Input: part model. Units: mm. Frame: model coordinates. A direction names the side the tool comes from. Round coordinates to 2 decimals unless told otherwise and drop trailing zeros. Loops run counter-clockwise (first coordinate to the right, second up) from the corner with the lowest first, then second, coordinate; pieces in that order, holes last. Notation, with made-up numbers: M -11.5,12.5 L 16.5,12.5 A31 cw 16.5,49.5 Z; hole C 41.5,25 d8. An arc over 180 degrees is marked long. Put each result on its own line as item: value. Start each with the question number.
1) Line query: probe 1 along Y at (x, z) = (0.7, -29); probe 2 along Y at (x, z) = (2.3, 20). Output: solid intervals per line, ascending.
2) Draft query along Y for faces 3 (the face through (1, -24, 0)), 4 (the face through (1.52, -27, -31.45)), 5 (the face through (1, 0, -32.5)), 6 (the face through (2.507, -12.307, 18.8)). Return one class per face: +Y half, -Y half, draft (parallel to the pull), parting line (faces both ways), or undercut.
3) Reachability of faces 1 (the face through (1, 6, 27.857)), 2 (the face through (7, 22.99, 29.05)) from +Z, -Z, +X, -X, +Y, -Y: full face, straight path, thin tool, end or side. Return the list, or none.
4) Section C-C on z = -1. Output: boundary loops of the cut face in (x, y), plus the area to 3 significant figures.
5) Section B-B on y = -10. Output: boundary loops of the cut face in (x, z).
6) Section D-D on z = -20. Output: boundary loops of the cut face in (x, y), plus the area to 3 significant figures.
7) Pin query (flat end, axial travel): pin 1 (1.6 mm diameter, centred on y = -9.5, z = 19, fed in from +X); pin 2 (1.8 mm diameter, centred on y = -19.5, z = 21.5, fed in from +X). Return the tip coordinate at first contact, or that it passes through.
from build123d import *
from build123d.topology import SkipClean

# Parameters (mm, degrees)
SKETCH1_W           = 65
SKETCH1_H           = 56
SKETCH1_W_2         = 55.714285714
SKETCH1_H_2         = 48
BOSS_EXTRUDE1_DEPTH = 3
BOSS_EXTRUDE2_DEPTH = 4
BOSS_EXTRUDE3_DEPTH = 3
SKETCH4_R           = 1.35
CUT_EXTRUDE1_DEPTH  = 44.084219849
FILLET1_R           = 3.5
SKETCH5_W           = 55.714285714
SKETCH5_H           = 10
BOSS_EXTRUDE4_DEPTH = 3
SKETCH6_R           = 1.3
CUT_EXTRUDE2_DEPTH  = 44.084219849
BOSS_EXTRUDE5_DEPTH = 3
SKETCH8_R           = 2.6
CUT_EXTRUDE3_DEPTH  = 1


with BuildPart() as part:
    # Sketch1 → Boss-Extrude1 (new body)
    with BuildSketch(Plane(origin=(0, 0, 0), x_dir=(0, 0, -1), z_dir=(1, 0, 0))):
        Rectangle(SKETCH1_W, SKETCH1_H)
        Rectangle(SKETCH1_W_2, SKETCH1_H_2, mode=Mode.SUBTRACT)
    extrude(amount=BOSS_EXTRUDE1_DEPTH)

    # Sketch2 → Boss-Extrude2 (add)
    with BuildSketch(Plane(origin=(3, 0, 0), x_dir=(0, 0, -1), z_dir=(1, 0, 0))):
        with BuildLine():
            ThreePointArc((-25.5, 24.5), (-31.474873734, 26.974873734), (-29, 21))
            Line((-29, 21), (-29, 23.15))
            ThreePointArc((-29, 23.15), (-29.954594155, 25.454594155), (-27.65, 24.5))
            Line((-27.65, 24.5), (-25.5, 24.5))
        make_face()
        with BuildLine():
            Line((-29, 23.15), (-29, 21))
            ThreePointArc((-29, 21), (-28.420576225, 21.048294901), (-27.857142857, 21.191846807))
            Line((-27.857142857, 21.191846807), (-27.857142857, 23.781405851))
            ThreePointArc((-27.857142857, 23.781405851), (-28.347160855, 23.318348169), (-29, 23.15))
        make_face()
        with BuildLine():
            Line((-27.857142857, 23.781405851), (-27.857142857, 21.191846807))
            ThreePointArc((-27.857142857, 21.191846807), (-26.302325383, 22.270078104), (-25.535898385, 24))
            Line((-25.535898385, 24), (-27.74600638, 24))
            ThreePointArc((-27.74600638, 24), (-27.796600962, 23.888174245), (-27.857142857, 23.781405851))
        make_face()
        with BuildLine():
            ThreePointArc((-25.535898385, 24), (-25.508986132, 24.249356481), (-25.5, 24.5))
            Line((-25.5, 24.5), (-27.65, 24.5))
            ThreePointArc((-27.65, 24.5), (-27.674218836, 24.245433101), (-27.74600638, 24))
            Line((-27.74600638, 24), (-25.535898385, 24))
        make_face()
        with BuildLine():
            Line((29, 23.15), (29, 21))
            ThreePointArc((29, 21), (31.474873734, 22.025126266), (32.5, 24.5))
            ThreePointArc((32.5, 24.5), (29, 28), (25.5, 24.5))
            Line((25.5, 24.5), (27.65, 24.5))
            ThreePointArc((27.65, 24.5), (29, 25.85), (30.35, 24.5))
            ThreePointArc((30.35, 24.5), (29.954594155, 23.545405845), (29, 23.15))
        make_face()
        with BuildLine():
            Line((27.65, 24.5), (25.5, 24.5))
            ThreePointArc((25.5, 24.5), (25.508986132, 24.249356481), (25.535898385, 24))
            Line((25.535898385, 24), (27.74600638, 24))
            ThreePointArc((27.74600638, 24), (27.674218836, 24.245433101), (27.65, 24.5))
        make_face()
        with BuildLine():
            ThreePointArc((25.535898385, 24), (26.302325383, 22.270078104), (27.857142857, 21.191846807))
            Line((27.857142857, 21.191846807), (27.857142857, 23.781405851))
            ThreePointArc((27.857142857, 23.781405851), (27.796600962, 23.888174245), (27.74600638, 24))
            Line((27.74600638, 24), (25.535898385, 24))
        make_face()
        with BuildLine():
            Line((27.857142857, 23.781405851), (27.857142857, 21.191846807))
            ThreePointArc((27.857142857, 21.191846807), (28.420576225, 21.048294901), (29, 21))
            Line((29, 21), (29, 23.15))
            ThreePointArc((29, 23.15), (28.347160855, 23.318348169), (27.857142857, 23.781405851))
        make_face()
        with BuildLine():
            Line((27.65, -24.5), (25.5, -24.5))
            ThreePointArc((25.5, -24.5), (29, -28), (32.5, -24.5))
            ThreePointArc((32.5, -24.5), (31.474873734, -22.025126266), (29, -21))
            Line((29, -21), (29, -23.15))
            ThreePointArc((29, -23.15), (29.954594155, -23.545405845), (30.35, -24.5))
            ThreePointArc((30.35, -24.5), (29, -25.85), (27.65, -24.5))
        make_face()
        with BuildLine():
            ThreePointArc((29, -21), (28.420576225, -21.048294901), (27.857142857, -21.191846807))
            Line((27.857142857, -21.191846807), (27.857142857, -23.781405851))
            ThreePointArc((27.857142857, -23.781405851), (28.347160855, -23.318348169), (29, -23.15))
            Line((29, -23.15), (29, -21))
        make_face()
        with BuildLine():
            ThreePointArc((27.857142857, -21.191846807), (26.302325383, -22.270078104), (25.535898385, -24))
            Line((25.535898385, -24), (27.74600638, -24))
            ThreePointArc((27.74600638, -24), (27.796600962, -23.888174245), (27.857142857, -23.781405851))
            Line((27.857142857, -23.781405851), (27.857142857, -21.191846807))
        make_face()
        with BuildLine():
            ThreePointArc((25.535898385, -24), (25.508986132, -24.249356481), (25.5, -24.5))
            Line((25.5, -24.5), (27.65, -24.5))
            ThreePointArc((27.65, -24.5), (27.674218836, -24.245433101), (27.74600638, -24))
            Line((27.74600638, -24), (25.535898385, -24))
        make_face()
        with BuildLine():
            ThreePointArc((-29, -21), (-31.474873734, -26.974873734), (-25.5, -24.5))
            Line((-25.5, -24.5), (-27.65, -24.5))
            ThreePointArc((-27.65, -24.5), (-29.954594155, -25.454594155), (-29, -23.15))
            Line((-29, -23.15), (-29, -21))
        make_face()
        with BuildLine():
            ThreePointArc((-27.857142857, -21.191846807), (-28.420576225, -21.048294901), (-29, -21))
            Line((-29, -21), (-29, -23.15))
            ThreePointArc((-29, -23.15), (-28.347160855, -23.318348169), (-27.857142857, -23.781405851))
            Line((-27.857142857, -23.781405851), (-27.857142857, -21.191846807))
        make_face()
        with BuildLine():
            Line((-27.74600638, -24), (-25.535898385, -24))
            ThreePointArc((-25.535898385, -24), (-26.302325383, -22.270078104), (-27.857142857, -21.191846807))
            Line((-27.857142857, -21.191846807), (-27.857142857, -23.781405851))
            ThreePointArc((-27.857142857, -23.781405851), (-27.796600962, -23.888174245), (-27.74600638, -24))
        make_face()
        with BuildLine():
            Line((-27.65, -24.5), (-25.5, -24.5))
            ThreePointArc((-25.5, -24.5), (-25.508986132, -24.249356481), (-25.535898385, -24))
            Line((-25.535898385, -24), (-27.74600638, -24))
            ThreePointArc((-27.74600638, -24), (-27.674218836, -24.245433101), (-27.65, -24.5))
        make_face()
    extrude(amount=BOSS_EXTRUDE2_DEPTH)

    # Sketch3 → Boss-Extrude3 (add)
    with SkipClean():  # the faces are left unmerged after this step: merging them gives an invalid solid
        with BuildSketch(Plane.ZY):
            with BuildLine():
                Line((-27.74600638, 24), (-27.857142857, 24))
                Line((-27.857142857, 24), (-27.857142857, 23.781405851))
                Line((-27.857142857, 23.781405851), (-27.857142857, 21.191846807))
                ThreePointArc((-27.857142857, 21.191846807), (-26.302325383, 22.270078104), (-25.535898385, 24))
                Line((-25.535898385, 24), (-27.74600638, 24))
            make_face()
            with BuildLine():
                Line((27.857142857, 21.191846807), (27.857142857, 23.781405851))
                Line((27.857142857, 23.781405851), (27.857142857, 24))
                Line((27.857142857, 24), (27.74600638, 24))
                Line((27.74600638, 24), (25.535898385, 24))
                ThreePointArc((25.535898385, 24), (26.302325383, 22.270078104), (27.857142857, 21.191846807))
            make_face()
            with BuildLine():
                Line((-27.857142857, -21.191846807), (-27.857142857, -23.781405851))
                Line((-27.857142857, -23.781405851), (-27.857142857, -24))
                Line((-27.857142857, -24), (-27.74600638, -24))
                Line((-27.74600638, -24), (-25.535898385, -24))
                ThreePointArc((-25.535898385, -24), (-26.302325383, -22.270078104), (-27.857142857, -21.191846807))
            make_face()
            with BuildLine():
                Line((27.857142857, -23.781405851), (27.857142857, -21.191846807))
                ThreePointArc((27.857142857, -21.191846807), (26.302325383, -22.270078104), (25.535898385, -24))
                Line((25.535898385, -24), (27.74600638, -24))
                Line((27.74600638, -24), (27.857142857, -24))
                Line((27.857142857, -24), (27.857142857, -23.781405851))
            make_face()
        extrude(amount=-BOSS_EXTRUDE3_DEPTH)

    # Sketch4 → Cut-Extrude1 (cut, through all)
    with BuildSketch(Plane(origin=(3, 0, 0), x_dir=(0, 0, -1), z_dir=(1, 0, 0))):
        with Locations((29, -24.5)):
            Circle(SKETCH4_R)
        with Locations((-29, -24.5)):
            Circle(SKETCH4_R)
        with Locations((29, 24.5)):
            Circle(SKETCH4_R)
        with Locations((-29, 24.5)):
            Circle(SKETCH4_R)
    extrude(amount=-CUT_EXTRUDE1_DEPTH, mode=Mode.SUBTRACT)

    # Fillet1
    fillet1_edges = [part.edges().sort_by_distance(p)[0] for p in [
        (1.5, -28, 32.5),
        (1.5, 28, 32.5),
        (1.5, -28, -32.5),
        (1.5, 28, -32.5),
    ]]
    fillet(fillet1_edges, radius=FILLET1_R)

    # Sketch5 → Boss-Extrude4 (add)
    with BuildSketch(Plane(origin=(3, 0, 0), x_dir=(0, 0, -1), z_dir=(1, 0, 0))):
        with Locations((0, -13)):
            Rectangle(SKETCH5_W, SKETCH5_H)
    extrude(amount=-BOSS_EXTRUDE4_DEPTH)

    # Sketch6 → Cut-Extrude2 (cut, through all)
    with SkipClean():  # the faces are left unmerged after this step: merging them gives an invalid solid
        with BuildSketch(Plane(origin=(3, 0, 0), x_dir=(0, 0, -1), z_dir=(1, 0, 0))):
            with Locations((-20, -10)):
                Circle(SKETCH6_R)
            with Locations((-20, -16)):
                Circle(SKETCH6_R)
            with Locations((20, -10)):
                Circle(SKETCH6_R)
            with Locations((20, -16)):
                Circle(SKETCH6_R)
        extrude(amount=-CUT_EXTRUDE2_DEPTH, mode=Mode.SUBTRACT)

    # Sketch7 → Boss-Extrude5 (add)
    with SkipClean():  # the faces are left unmerged after this step: merging them gives an invalid solid
        with BuildSketch(Plane(origin=(3, 0, 0), x_dir=(0, 0, -1), z_dir=(1, 0, 0))):
            with BuildLine():
                Line((-23.806573262, -8), (-16.193426738, -8))
                ThreePointArc((-16.193426738, -8), (-20, -5.7), (-23.806573262, -8))
            make_face()
            with BuildLine():
                Line((16.193426738, -8), (23.806573262, -8))
                ThreePointArc((23.806573262, -8), (20, -5.7), (16.193426738, -8))
            make_face()
            with BuildLine():
                ThreePointArc((-23.806573262, -18), (-20, -20.3), (-16.193426738, -18))
                Line((-16.193426738, -18), (-23.806573262, -18))
            make_face()
            with BuildLine():
                Line((23.806573262, -18), (16.193426738, -18))
                ThreePointArc((16.193426738, -18), (20, -20.3), (23.806573262, -18))
            make_face()
        extrude(amount=-BOSS_EXTRUDE5_DEPTH)

    # Sketch8 → Cut-Extrude3 (cut)
    with SkipClean():  # the faces are left unmerged after this step: merging them gives an invalid solid
        with BuildSketch(Plane(origin=(3, 0, 0), x_dir=(0, 0, -1), z_dir=(1, 0, 0))):
            with Locations((-20, -10)):
                Circle(SKETCH8_R)
            with Locations((-20, -16)):
                Circle(SKETCH8_R)
            with Locations((20, -10)):
                Circle(SKETCH8_R)
            with Locations((20, -16)):
                Circle(SKETCH8_R)
        extrude(amount=-CUT_EXTRUDE3_DEPTH, mode=Mode.SUBTRACT)


solid = part.part
Geometry results:
1. probe 1: y = -28 to -25.85, -23.15 to 23.15, 25.85 to 28
1. probe 2: y = -28 to -24, -20.3 to -18.6, -13.4 to -12.6, -7.4 to -5.7, 24 to 28
2. face 3: undercut
2. face 4: -Y half
2. face 5: draft
2. face 6: undercut
3. face 1: +X, -X
3. face 2: +Z, -Z, +X, +Y, -Y
4. outline: M 0,-28 L 3,-28 L 3,-24 L 0,-24 Z; M 0,-18 L 3,-18 L 3,-8 L 0,-8 Z; M 0,24 L 3,24 L 3,28 L 0,28 Z
4. area: 54.0 mm²
5. outline: M 0,-32.5 L 3,-32.5 L 3,-22.6 L 2,-22.6 L 2,-21.3 L 0,-21.3 Z; M 0,-18.7 L 2,-18.7 L 2,-17.4 L 3,-17.4 L 3,17.4 L 2,17.4 L 2,18.7 L 0,18.7 Z; M 0,21.3 L 2,21.3 L 2,22.6 L 3,22.6 L 3,32.5 L 0,32.5 Z
6. outline: M 0,-28 L 3,-28 L 3,-24 L 0,-24 Z; M 0,-20.3 L 3,-20.3 L 3,-18.6 L 2,-18.6 L 2,-17.3 L 0,-17.3 Z; M 0,-14.7 L 2,-14.7 L 2,-13.4 L 3,-13.4 L 3,-12.6 L 2,-12.6 L 2,-11.3 L 0,-11.3 Z; M 0,-8.7 L 2,-8.7 L 2,-7.4 L 3,-7.4 L 3,-5.7 L 0,-5.7 Z; M 0,24 L 3,24 L 3,28 L 0,28 Z
6. area: 47.0 mm²
7. pin 1: stops at x = 2
7. pin 2: stops at x = 3
